For this review, take the finished solid that the model builds, in its own axes (mm). Face numbers are marked on the shaded views. Round coordinates to 2 decimals unless told otherwise and drop trailing zeros. Order: outer loops, then holes, each group sorted by start corner. A loop starts at its lowest first (then second) coordinate and runs counter-clockwise, first axis right, second up. Notation, with made-up numbers: (-17, 47) -> (31, 47) arc R23 cw to (31, 83) -> close; hole circle Ø5 at (-33, -36.75). An arc over 180 degrees is marked (long way). Put each result on its own line as item: value. Start each with the question number.
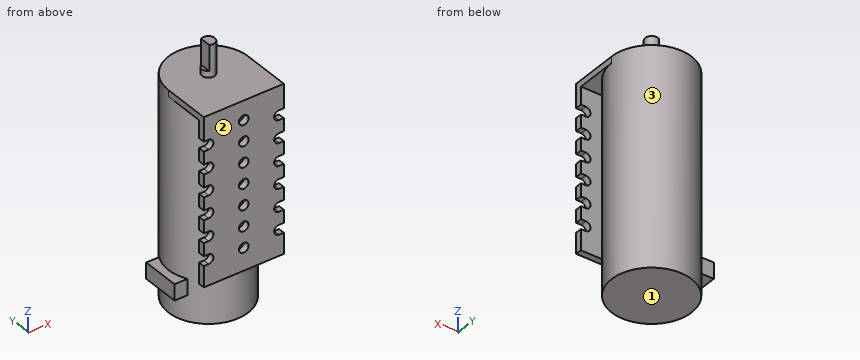
```python
from build123d import *

# Parameters (mm, degrees)
SKETCH1_R           = 12.5
BOSS_EXTRUDE1_DEPTH = 68
SKETCH3_R           = 2
BOSS_EXTRUDE3_DEPTH = 2
BOSS_EXTRUDE2_DEPTH = 8
BOSS_EXTRUDE4_DEPTH = 2
SKETCH5_W           = 25
SKETCH5_H           = 2
BOSS_EXTRUDE5_DEPTH = 50
SKETCH6_R           = 1.5
CUT_EXTRUDE1_DEPTH  = 2
SKETCH7_W           = 5
SKETCH7_H           = 12
BOSS_EXTRUDE6_DEPTH = 15


with BuildPart() as part:
    # Sketch1 → Boss-Extrude1 (new body)
    with BuildSketch(Plane.XY):
        Circle(SKETCH1_R)
    extrude(amount=-BOSS_EXTRUDE1_DEPTH)

    # Sketch3 → Boss-Extrude3 (add)
    with BuildSketch(Plane.XY):
        Circle(SKETCH3_R)
    extrude(amount=BOSS_EXTRUDE3_DEPTH)

    # Sketch2 → Boss-Extrude2 (add)
    with BuildSketch(Plane.XY.offset(2)):
        with BuildLine():
            Line((-1, 1.732050808), (-1, -1.732050808))
            ThreePointArc((-1, -1.732050808), (2, 0), (-1, 1.732050808))
        make_face()
    extrude(amount=BOSS_EXTRUDE2_DEPTH)

    # Sketch4 → Boss-Extrude4 (add)
    with BuildSketch(Plane.XY):
        with BuildLine():
            Line((-12.5, 0), (-12.5, -15))
            Line((-12.5, -15), (12.5, -15))
            Line((12.5, -15), (12.5, 0))
            ThreePointArc((12.5, 0), (0, -12.5), (-12.5, 0))
        make_face()
    extrude(amount=-BOSS_EXTRUDE4_DEPTH)

    # Sketch5 → Boss-Extrude5 (add)
    with BuildSketch(Plane(origin=(0, 0, -2), x_dir=(-1, 0, 0), z_dir=(0, 0, -1))):
        with Locations((0, -14)):
            Rectangle(SKETCH5_W, SKETCH5_H)
    extrude(amount=BOSS_EXTRUDE5_DEPTH)

    # Sketch6 → Cut-Extrude1 (cut)
    with BuildSketch(Plane.XZ.offset(15)):
        with Locations(Location((0, -6, 0), (0, 0, 270))):
            Circle(SKETCH6_R)
        with Locations(Location((0, -12.5, 0), (0, 0, 270))):
            Circle(SKETCH6_R)
        with Locations(Location((0, -19, 0), (0, 0, 270))):
            Circle(SKETCH6_R)
        with Locations(Location((0, -25.5, 0), (0, 0, 270))):
            Circle(SKETCH6_R)
        with Locations(Location((0, -32, 0), (0, 0, 270))):
            Circle(SKETCH6_R)
        with Locations(Location((0, -38.5, 0), (0, 0, 270))):
            Circle(SKETCH6_R)
        with Locations(Location((0, -45, 0), (0, 0, 270))):
            Circle(SKETCH6_R)
        with BuildLine():
            Line((-11, -7.5), (-12.5, -7.5))
            Line((-12.5, -7.5), (-12.5, -10.5))
            Line((-12.5, -10.5), (-11, -10.5))
            ThreePointArc((-11, -10.5), (-9.5, -9), (-11, -7.5))
        make_face()
        with BuildLine():
            Line((-11, -14.5), (-12.5, -14.5))
            Line((-12.5, -14.5), (-12.5, -17.5))
            Line((-12.5, -17.5), (-11, -17.5))
            ThreePointArc((-11, -17.5), (-9.5, -16), (-11, -14.5))
        make_face()
        with BuildLine():
            Line((-11, -21.5), (-12.5, -21.5))
            Line((-12.5, -21.5), (-12.5, -24.5))
            Line((-12.5, -24.5), (-11, -24.5))
            ThreePointArc((-11, -24.5), (-9.5, -23), (-11, -21.5))
        make_face()
        with BuildLine():
            Line((-11, -28.5), (-12.5, -28.5))
            Line((-12.5, -28.5), (-12.5, -31.5))
            Line((-12.5, -31.5), (-11, -31.5))
            ThreePointArc((-11, -31.5), (-9.5, -30), (-11, -28.5))
        make_face()
        with BuildLine():
            Line((-11, -35.5), (-12.5, -35.5))
            Line((-12.5, -35.5), (-12.5, -38.5))
            Line((-12.5, -38.5), (-11, -38.5))
            ThreePointArc((-11, -38.5), (-9.5, -37), (-11, -35.5))
        make_face()
        with BuildLine():
            Line((-11, -42.5), (-12.5, -42.5))
            Line((-12.5, -42.5), (-12.5, -45.5))
            Line((-12.5, -45.5), (-11, -45.5))
            ThreePointArc((-11, -45.5), (-9.5, -44), (-11, -42.5))
        make_face()
        with BuildLine():
            Line((11, -45.5), (12.5, -45.5))
            Line((12.5, -45.5), (12.5, -42.5))
            Line((12.5, -42.5), (11, -42.5))
            ThreePointArc((11, -42.5), (9.5, -44), (11, -45.5))
        make_face()
        with BuildLine():
            Line((11, -38.5), (12.5, -38.5))
            Line((12.5, -38.5), (12.5, -35.5))
            Line((12.5, -35.5), (11, -35.5))
            ThreePointArc((11, -35.5), (9.5, -37), (11, -38.5))
        make_face()
        with BuildLine():
            Line((11, -31.5), (12.5, -31.5))
            Line((12.5, -31.5), (12.5, -28.5))
            Line((12.5, -28.5), (11, -28.5))
            ThreePointArc((11, -28.5), (9.5, -30), (11, -31.5))
        make_face()
        with BuildLine():
            Line((11, -24.5), (12.5, -24.5))
            Line((12.5, -24.5), (12.5, -21.5))
            Line((12.5, -21.5), (11, -21.5))
            ThreePointArc((11, -21.5), (9.5, -23), (11, -24.5))
        make_face()
        with BuildLine():
            Line((11, -17.5), (12.5, -17.5))
            Line((12.5, -17.5), (12.5, -14.5))
            Line((12.5, -14.5), (11, -14.5))
            ThreePointArc((11, -14.5), (9.5, -16), (11, -17.5))
        make_face()
        with BuildLine():
            Line((11, -7.5), (12.5, -7.5))
            Line((12.5, -7.5), (12.5, -10.5))
            Line((12.5, -10.5), (11, -10.5))
            ThreePointArc((11, -10.5), (9.5, -9), (11, -7.5))
        make_face()
    extrude(amount=-CUT_EXTRUDE1_DEPTH, mode=Mode.SUBTRACT)

    # Sketch7 → Boss-Extrude6 (add)
    with BuildSketch(Plane(origin=(0, 0, 0), x_dir=(0, 0, -1), z_dir=(1, 0, 0))):
        with Locations((57.5, 0)):
            Rectangle(SKETCH7_W, SKETCH7_H)
    extrude(amount=-BOSS_EXTRUDE6_DEPTH)


solid = part.part
```
Item 1: Consider section C-C, the plane y = -3. Write out the cut boundary in (x, z).
Item 2: Consider section A-A, the plane z = -12.5. Write out the cut boundary in (x, y).
Item 3: Consider section B-B, the plane z = -47.5. Write out the cut boundary in (x, y), plus the area to 3 significant figures.
Item 4: Consider section D-D, the plane z = -23. Write out the cut boundary in (x, y), plus the area to 3 significant figures.
Item 5: Mouldability with a two-part tool opening along Y and no side actions: class the marked faces 1, 2 and 3 as +Y half, -Y half, draft (parallel to the pull), parting line (faces both ways), or undercut.
Item 6: For L1, parallel to Y at x = 0.5, z = -10; L2, parallel to X at y = -13.4, z = -6; L3, parallel to Y at x = 9.5, z = -18.5, list the stretches that pass through material, from the lowest coordinate up.
Item 7: Insertion check: pin 1 Ø0.8 at (x, y) = (-12, -14) entering from -Z; pin 2 Ø1.6 at (y, z) = (-14, -40.5) entering from -X; pin 3 Ø10 at (x, y) = (-12, -4.5) entering from +Z. Each pin has a flat end and moves straight along its axis. Give the tip position at first contact, or say it passes through.
Evaluation:
1. outline: (-15, -60) -> (-12.13, -60) -> (-12.13, -68) -> (12.13, -68) -> (12.13, -2) -> (12.5, -2) -> (12.5, 0) -> (-12.5, 0) -> (-12.5, -2) -> (-12.13, -2) -> (-12.13, -55) -> (-15, -55) -> close
2. outline: (-12.5, -15) -> (-1.5, -15) -> (-1.5, -13) -> (-12.5, -13) -> close; circle Ø25 at (0, 0); (1.5, -15) -> (12.5, -15) -> (12.5, -13) -> (1.5, -13) -> close
3. outline: (-12.5, -15) -> (12.5, -15) -> (12.5, -13) -> (-12.5, -13) -> close; circle Ø25 at (0, 0)
3. area: 541 mm^2
4. outline: circle Ø25 at (0, 0); (-9.5, -15) -> (9.5, -15) -> (9.5, -13) -> (-9.5, -13) -> close
4. area: 529 mm^2
5. face 1: draft
5. face 2: -Y half
5. face 3: undercut
6. L1: y = -15 to -13, -12.49 to 12.49
6. L2: x = -12.5 to -1.5, 1.5 to 12.5
6. L3: y = -15 to -13, -8.12 to 8.12
7. pin 1: stops at z = -52
7. pin 2: stops at x = -12.5
7. pin 3: stops at z = 0
